Build history of the part. All positions in model axes, mm. A direction names the side the tool comes from. Give positions to 0.01 mm unless a question says otherwise; leave off trailing zeros. Loops run counter-clockwise (first coordinate to the right, second up) from the corner with the lowest first, then second, coordinate; pieces in that order, holes last. Notation, with made-up numbers: (36.25, 74) -> (53.25, 74) arc R26 ccw to (53.25, 98) -> close; hole circle Ø4 at (52.5, 40). An arc over 180 degrees is marked (long way). Answer as a JSON object with one key per item and string values. Group by question number.
Q1. Band-saw the part on A-A, the plane y = 0. Write the cut outline in (x, z).
Q2. Band-saw the part on B-B, the plane x = 2. Write the cut outline in (y, z), plus the area to 3 significant figures.
Q3. Two-plate mould, pull along X, no slides. Class faces 3 (the cylindrical face through (-27.83, 11, 1.52)), 4 (the flat face through (-34.03, 0, -1)), 5 (the flat face through (-29, 12, 3)): pulls with the +X half, pulls with the -X half, needs draft (parallel to the pull), parting line crosses it, or undercut.
Q4. Tool access for faces 1 (the flat face through (33.97, 0, -1)), 2 (the cylindrical face through (-27.83, -12, 1.52)): list every direction of +Z, -Z, +X, -X, +Y, -Y with a clear straight run to the whole face (end or side of a thin tool).
Q5. Band-saw the part on C-C, the plane z = 1.95. Write the cut outline in (x, y).
Q6. Wall check: probe 1 along Z at (x, y) = (-12, 6); probe 2 along Y at (x, z) = (30, 0.3); probe 3 along X at (y, z) = (11, 0.9). Give the ranges that are in metal, low to high. Write a range as from..to.
Q7. Drop a flat-ended pin along its axis: pin 1 (8 mm diameter, centred on x = 1.5, y = -11, fed in from +Z). Give the stop position or say it passes through.
from build123d import *

# Parameters (mm, degrees)
F0_R          = 1.3
F1_DEPTH      = 3
F1_DEPTH_BACK = 1.5
F0_W          = 68
F0_H          = 32
F2_DEPTH      = 1.5


with BuildPart() as f1:
    # F0 (on Top) → F1 (new body, two sides)
    with BuildSketch(Plane.XY) as f1_sk:
        with Locations((-29.0296536804, -11.5017628863)):
            Circle(F0_R)
    extrude(amount=F1_DEPTH)
    extrude(f1_sk.sketch, amount=-F1_DEPTH_BACK)



with BuildPart() as f1b:
    # F0 (on Top) → F1, piece 2 (new body, two sides)
    with BuildSketch(Plane.XY) as f1_2_sk:
        with Locations((-29.0296536804, 11.4982371137)):
            Circle(F0_R)
    extrude(amount=F1_DEPTH)
    extrude(f1_2_sk.sketch, amount=-F1_DEPTH_BACK)


with BuildPart() as f1c:
    # F0 (on Top) → F1, piece 3 (new body, two sides)
    with BuildSketch(Plane.XY) as f1_3_sk:
        with Locations((28.9703463196, 11.4982371137)):
            Circle(F0_R)
    extrude(amount=F1_DEPTH)
    extrude(f1_3_sk.sketch, amount=-F1_DEPTH_BACK)


with BuildPart() as f1d:
    # F0 (on Top) → F1, piece 4 (new body, two sides)
    with BuildSketch(Plane.XY) as f1_4_sk:
        with Locations((28.9703463196, -11.5017628863)):
            Circle(F0_R)
    extrude(amount=F1_DEPTH)
    extrude(f1_4_sk.sketch, amount=-F1_DEPTH_BACK)


with BuildPart() as f1_1:
    add(f1.part)

    add(f1b.part)  # F2 merges F1b

    add(f1c.part)  # F2 merges F1c

    add(f1d.part)  # F2 merges F1d
    # F0 (on Top) → F2 (join)
    with BuildSketch(Plane.XY):
        with Locations((-0.0296536804, -0.0017628863)):
            Rectangle(F0_W, F0_H)
        with Locations((-29.0296536804, -11.5017628863)):
            Circle(F0_R, mode=Mode.SUBTRACT)
        with Locations((28.9703463196, -11.5017628863)):
            Circle(F0_R, mode=Mode.SUBTRACT)
        with Locations((-29.0296536804, 11.4982371137)):
            Circle(F0_R, mode=Mode.SUBTRACT)
        with Locations((28.9703463196, 11.4982371137)):
            Circle(F0_R, mode=Mode.SUBTRACT)
    extrude(amount=-F2_DEPTH)


solid = f1_1.part
Worked answers:
{
 "1": {"outline": "(-34.03, -1.5) -> (33.97, -1.5) -> (33.97, 0) -> (-34.03, 0) -> close"},
 "2": {"outline": "(-16, -1.5) -> (16, -1.5) -> (16, 0) -> (-16, 0) -> close", "area": "48.0 mm2"},
 "3": {"face 3": "undercut", "face 4": "pulls with the -X half", "face 5": "needs draft"},
 "4": {"face 1": "+Z, -Z, +X, +Y, -Y", "face 2": "+Z"},
 "5": {"outline": "circle Ø2.6 at (-29.03, -11.5); circle Ø2.6 at (-29.03, 11.5); circle Ø2.6 at (28.97, -11.5); circle Ø2.6 at (28.97, 11.5)"},
 "6": {"probe 1": "-1.5..0", "probe 2": "-12.3..-10.71, 10.7..12.29", "probe 3": "-30.23..-27.83, 27.77..30.17"},
 "7": {"pin 1": "z = 0"}
}
